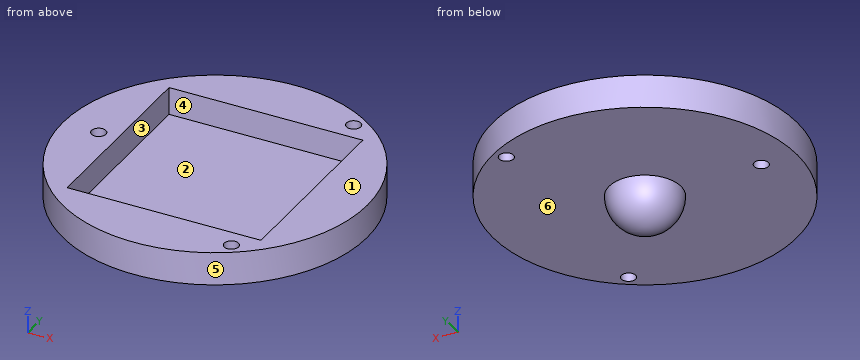
from build123d import *

# Parameters (mm, degrees)
SKETCH1_R            = 27.5
SKETCH1_W            = 37
SKETCH1_H            = 37
SKETCH1_W_2          = 35
SKETCH1_H_2          = 35
BOSS_EXTRUDE1_DEPTH  = 6
SKETCH1_3_W          = 35
SKETCH1_3_H          = 35
BOSS_EXTRUDE2_DEPTH  = 1
M2_CLEARANCE_HOLE1_D = 2.6


with BuildPart() as part:
    # Sketch1 → Boss-Extrude1 (new body)
    # profile 1 of 2: a face of its own
    with BuildSketch(Plane.XY):
        Circle(SKETCH1_R)
        Rectangle(SKETCH1_W, SKETCH1_H, mode=Mode.SUBTRACT)
    # profile 2 of 2: a face of its own
    with BuildSketch(Plane.XY):
        Rectangle(SKETCH1_W, SKETCH1_H)
        Rectangle(SKETCH1_W_2, SKETCH1_H_2, mode=Mode.SUBTRACT)
    extrude(amount=BOSS_EXTRUDE1_DEPTH)

    # Sketch1_3 → Boss-Extrude2 (add)
    with BuildSketch(Plane.XY):
        Rectangle(SKETCH1_3_W, SKETCH1_3_H)
    extrude(amount=BOSS_EXTRUDE2_DEPTH)

    # Sketch2 → Revolve1 (revolve)
    with BuildSketch(Plane(origin=(0, 0, 0), x_dir=(1, 0, 0), z_dir=(0, 1, 0)), mode=Mode.PRIVATE) as revolve1_sk:
        with BuildLine():
            Line((0, 6.5), (0, 0))
            Line((0, 0), (-6.5, 0))
            ThreePointArc((-6.5, 0), (-4.596194078, 4.596194078), (0, 6.5))
        make_face()
    revolve(revolve1_sk.sketch.rotate(Axis((0, 0, -15), (0, 0, 1)), 180), axis=Axis((0, 0, -15), (0, 0, 1)))

    # M2 Clearance Hole1 (through all)
    with Locations(Plane.XY.offset(6)):
        with Locations((-21, 0), (14, -21), (14, 21)):
            Hole(M2_CLEARANCE_HOLE1_D / 2)


solid = part.part
Here's how the part is built. I have some questions about the finished solid (model axes, mm). Face numbers are marked on the shaded views. A direction names the side the tool comes from. Coordinates: 2 decimals unless noted, no trailing zeros. Write each loop counter-clockwise with the first axis right and the second up, starting at its lowest first coordinate (ties: lowest second). Pieces come first, ordered by that corner, then holes.
1) If we section it at D-D (y = 11.5): List the corners of the cut face in (x, z) for me, plus the area to 3 significant figures.
Filled in:
outline: (-24.98, 0) - (24.98, 0) - (24.98, 6) - (17.5, 6) - (17.5, 1) - (-17.5, 1) - (-17.5, 6) - (-24.98, 6) - close
area: 125 mm2
2) If we section it at B-B (z = 1.75): List the corners of the cut face in (x, y) for me.
Filled in:
outline: circle Ø55 at (0, 0); hole circle Ø2.6 at (-21, 0); hole (-17.5, -17.5) - (17.5, -17.5) - (17.5, 17.5) - (-17.5, 17.5) - close; hole circle Ø2.6 at (14, -21); hole circle Ø2.6 at (14, 21)
3) If we section it at A-A (y = 0): List the corners of the cut face in (x, z) for me, plus the area to 3 significant figures.
Filled in:
outline: (-27.5, 0) - (-22.3, 0) - (-22.3, 6) - (-27.5, 6) - close; (-19.7, 0) - (-6.5, 0) arc R6.5 ccw to (6.5, 0) - (27.5, 0) - (27.5, 6) - (17.5, 6) - (17.5, 1) - (-17.5, 1) - (-17.5, 6) - (-19.7, 6) - close
area: 206 mm2
4) Thinking about a two-plate mould opening in X: for the marked faces 3, 4, 5 and 6, which applies, +X half, -X half, draft (parallel to the pull), parting line (faces both ways), or undercut?
Filled in:
face 3: undercut
face 4: undercut
face 5: parting line
face 6: draft
5) If we section it at C-C (x = -21): List the corners of the cut face in (y, z) for me, plus the area to 3 significant figures.
Filled in:
outline: (-17.76, 0) - (-1.3, 0) - (-1.3, 6) - (-17.76, 6) - close; (1.3, 0) - (17.76, 0) - (17.76, 6) - (1.3, 6) - close
area: 197 mm2
6) If I drill on line 1 (Y direction, x = 14, z = 4.7); line 2 (X direction, y = -1.5, z = 2.25); line 3 (Z direction, x = 11.5, y = 16.5), over which ranges is the centre line in solid material (lowest first)?
Filled in:
line 1: y = -23.67 to -22.3, -19.7 to -17.5, 17.5 to 19.7, 22.3 to 23.67
line 2: x = -27.46 to -17.5, 17.5 to 27.46
line 3: z = 0 to 1
7) Which directions (+Z, -Z, +X, -X, +Y, -Y) give clear straight access to the entire face, cutting with the end or side of a thin tool? Please do the marked faces 1 and 2.
Filled in:
face 1: +Z, +X, -X, +Y, -Y
face 2: +Z
8) I'm going to push flat-ended pins straight in: pin 1 (2.5 mm diameter, centred on x = 14, y = 21, fed in from +Z); pin 2 (4 mm diameter, centred on y = -3, z = 2.5, fed in from +X); pin 3 (17.5 mm diameter, centred on x = 1.5, y = -8, fed in from +Z); pin 4 (2.5 mm diameter, centred on x = 0, z = 3.5, fed in from -Y). Where does each tip first touch, or does it pass through?
Filled in:
pin 1: passes through
pin 2: stops at x = 27.48
pin 3: stops at z = 1
pin 4: stops at y = -27.5
